Can you work these out from the model? Positions are in its coordinate system, mm. Coordinates: 2 decimals unless noted, no trailing zeros. Write each loop counter-clockwise with the first axis right and the second up, starting at its lowest first coordinate (ties: lowest second). Pieces come first, ordered by that corner, then holes.
```python
from build123d import *

# Parameters (mm, degrees)
F0_W           = 101.6
F0_H           = 50.8
F1_DEPTH       = 152.4
F3_D           = 13.49248
F3_CSINK_D     = 23.8252
F3_CSINK_ANGLE = 82
F4_R           = 6.35
F5_SIZE        = 0.8128


with BuildPart() as f1:
    # F0 (on Front) → F1 (new body, symmetric)
    with BuildSketch(Plane.XZ):
        Rectangle(F0_W, F0_H)
    extrude(amount=F1_DEPTH, both=True)

    # F3 (through all)
    with Locations(Plane.XY.offset(25.4)):
        with Locations((-31.75, 133.35), (31.75, 133.35), (31.75, -133.35), (-31.75, -133.35)):
            CounterSinkHole(F3_D / 2, F3_CSINK_D / 2, counter_sink_angle=F3_CSINK_ANGLE)

    # F4
    f4_edges = [f1.edges().sort_by_distance(p)[0] for p in [
        (50.8, -152.4, 0),
        (50.8, 152.4, 0),
        (-50.8, -152.4, 0),
        (-50.8, 152.4, 0),
    ]]
    fillet(f4_edges, radius=F4_R)

    # F5
    f5_edges = [f1.edges().sort_by_distance(p)[0] for p in [
        (0, 152.4, 25.4),
        (50.8, 0, 25.4),
        (0, -152.4, 25.4),
        (-50.8, 0, 25.4),
        (-50.8, 0, -25.4),
        (-48.940128, 150.540128, -25.4),
        (-48.940128, -150.540128, -25.4),
        (0, 152.4, -25.4),
        (0, -152.4, -25.4),
        (48.940128, 150.540128, -25.4),
        (48.940128, -150.540128, -25.4),
        (50.8, 0, -25.4),
        (-38.49624, 133.35, -25.4),
        (25.00376, 133.35, -25.4),
        (-38.49624, -133.35, -25.4),
        (25.00376, -133.35, -25.4),
    ]]
    chamfer(f5_edges, length=F5_SIZE)


solid = f1.part
```
1. I'm going to push flat-ended pins straight in: P1, Ø17.5, axis at x = -31.75, y = -133.35, coming from the +Z side; P2, Ø21.5, axis at x = 31.75, y = 133.35, coming from the +Z side. Where does each tip first touch, or does it pass through?
2. If I drill on L1, parallel to X at y = -133.35, z = -5.5; L2, parallel to Y at x = -31.75, z = -12.5; L3, parallel to Y at x = -23.5, z = 23.5, over which ranges is the centre line in solid material (lowest first)?
3. If we section it at A-A, the plane x = -31.75: List the corners of the cut face in (y, z) for me, plus the area to 3 significant figures.
4. If we section it at B-B, the plane z = -20.5: List the corners of the cut face in (x, y) for me, plus the area to 3 significant figures.
5. If we section it at C-C, the plane y = -133.35: List the corners of the cut face in (x, z) for me.
6. We'd pull the mould along X, two halves only. Please class faces 1 (the face through (-1, -2, -25.4)), 2 (the face through (33.212, 126.764, -2.874)), 3 (the face through (-48.99, 150.49, 0.34)): released by +X, released by -X, zero draft, split by the parting line, or undercut.
Answers:
1. P1: stops at z = 21.76
1. P2: stops at z = 24.06
2. L1: x = -50.8 to -38.5, -25 to 25, 38.5 to 50.8
2. L2: y = -152.4 to -140.1, -126.6 to 126.6, 140.1 to 152.4
2. L3: y = -152.4 to -139.45, -127.25 to 127.25, 139.45 to 152.4
3. outline: (-152.4, -24.59) - (-151.59, -25.4) - (-140.91, -25.4) - (-140.1, -24.59) - (-140.1, 19.46) - (-145.26, 25.4) - (-151.59, 25.4) - (-152.4, 24.59) - close; (-126.6, -24.59) - (-125.79, -25.4) - (125.79, -25.4) - (126.6, -24.59) - (126.6, 19.46) - (121.44, 25.4) - (-121.44, 25.4) - (-126.6, 19.46) - close; (140.1, -24.59) - (140.91, -25.4) - (151.59, -25.4) - (152.4, -24.59) - (152.4, 24.59) - (151.59, 25.4) - (145.26, 25.4) - (140.1, 19.46) - close
3. area: 14,000 mm2
4. outline: (-50.8, -146.05) arc R6.35 ccw to (-44.45, -152.4) - (44.45, -152.4) arc R6.35 ccw to (50.8, -146.05) - (50.8, 146.05) arc R6.35 ccw to (44.45, 152.4) - (-44.45, 152.4) arc R6.35 ccw to (-50.8, 146.05) - close; hole circle Ø13.49 at (-31.75, -133.35); hole circle Ø13.49 at (-31.75, 133.35); hole circle Ø13.49 at (31.75, -133.35); hole circle Ø13.49 at (31.75, 133.35)
4. area: 30,400 mm2
5. outline: (-50.8, -24.59) - (-49.99, -25.4) - (-39.31, -25.4) - (-38.5, -24.59) - (-38.5, 19.46) - (-43.66, 25.4) - (-49.99, 25.4) - (-50.8, 24.59) - close; (-25, -24.59) - (-24.19, -25.4) - (24.19, -25.4) - (25, -24.59) - (25, 19.46) - (19.84, 25.4) - (-19.84, 25.4) - (-25, 19.46) - close; (38.5, -24.59) - (39.31, -25.4) - (49.99, -25.4) - (50.8, -24.59) - (50.8, 24.59) - (49.99, 25.4) - (43.66, 25.4) - (38.5, 19.46) - close
6. face 1: zero draft
6. face 2: undercut
6. face 3: released by -X
